Autodesk Inventor part; units mm, degrees
ref_plane "YZ Plane" through (0, 0, 0) normal (1, 0, 0) x (0, 1, 0)
ref_plane "XZ Plane" through (0, 0, 0) normal (0, 1, 0) x (-1, 0, 0)
ref_plane "XY Plane" through (0, 0, 0) normal (0, 0, 1) x (1, 0, 0)
sketch "Эскиз1" plane through (0, 0, 0) normal (0, 0, 1) x (1, 0, 0)
  line L0 (-8.89, 0) -> (53.01, 0)
  line L1 (53.01, 0) -> (53.01, 35.55)
  line L2 (53.01, 35.55) -> (-8.89, 35.55)
  line L3 (-8.89, 35.55) -> (-8.89, 0)
  circle A0 centre (15.24, 22.86) radius 0.405
  circle A1 centre (17.78, 22.86) radius 0.405
  circle A2 centre (20.32, 22.86) radius 0.405
  circle A3 centre (22.86, 22.86) radius 0.405
  circle A4 centre (25.4, 22.86) radius 0.405
  circle A5 centre (27.94, 22.86) radius 0.405
  circle A6 centre (37.62, 19.41) radius 0.405
  circle A7 centre (40.16, 19.41) radius 0.405
  circle A8 centre (0.1, 31.17) radius 0.65
  circle A9 centre (-4.9, 31.17) radius 0.65
  circle A10 centre (1.27, 20.32) radius 0.51
  circle A11 centre (-1.27, 20.32) radius 0.51
  circle A12 centre (-3.81, 20.32) radius 0.51
  circle A13 centre (-6.35, 20.32) radius 0.51
  circle A14 centre (48.26, 25.4) radius 0.65
  circle A15 centre (48.26, 30.4) radius 0.65
  circle A16 centre (9.33, 4.16) radius 0.51
  circle A17 centre (11.87, 4.16) radius 0.51
  circle A18 centre (14.41, 4.16) radius 0.51
  circle A19 centre (16.95, 4.16) radius 0.51
  circle A20 centre (19.49, 4.16) radius 0.51
  circle A21 centre (39.37, 15.24) radius 0.51
  circle A22 centre (41.91, 15.24) radius 0.51
  circle A23 centre (49.59, 7.57) radius 0.65
  circle A24 centre (49.59, 12.57) radius 0.65
  circle A25 centre (46.2, 8.43) radius 0.7
  circle A26 centre (46.2, 11.93) radius 0.7
  circle A27 centre (12.7, 24.13) radius 0.3
  circle A28 centre (5.08, 26.67) radius 0.3
  circle A29 centre (5.08, 24.13) radius 0.3
  circle A30 centre (12.7, 26.67) radius 0.3
  circle A31 centre (5.08, 31.75) radius 0.3
  circle A32 centre (5.08, 29.21) radius 0.3
  circle A33 centre (12.7, 29.21) radius 0.3
  circle A34 centre (12.7, 31.75) radius 0.3
  circle A35 centre (33.02, 25.4) radius 0.5
  circle A36 centre (33.02, 27.94) radius 0.5
  circle A37 centre (33.02, 22.86) radius 0.5
  circle A38 centre (-5.9225, 7.3465) radius 1.5
  circle A39 centre (39.37, 2.54) radius 1.5
  circle A40 centre (46.99, 19.05) radius 1.5
  circle A41 centre (6.0563, 20.3433) radius 1.5
  circle A42 centre (17.1236, 18.9948) radius 0.4
  circle A43 centre (17.0778, 15.6995) radius 0.4
extrude "OmniBot_motor_driver.brdКонтур" add sketch "Эскиз1" along normal blind 1.6
properties part number "000.006.001 - Плата"
Read the model definition and answer for the solid it produces. Units are mm, in the model's axes. Give positions to 0.01 mm unless a question says otherwise; leave off trailing zeros. Write each loop counter-clockwise with the first axis right and the second up, starting at its lowest first coordinate (ties: lowest second). Pieces come first, ordered by that corner, then holes. Notation, with made-up numbers: M -26,-18 L 14,-18 A10 cw 14,-8 Z; hole C -19,16.5 d11. An arc over 180 degrees is marked long. Put each result on its own line as item: value. Start each with the question number.
1. Consider line 1 along Y through (x, z) = (12.7, 0.9); line 2 along Y through (x, z) = (49.5, 0.95); line 3 along Y through (x, z) = (37.62, 1.15) (3 decimals). Determine where each line is inside the solid, lowest interval first.
2. For a pull along X with two mould halves and no side action, classify faces 1 (the cylindrical face through (48.42, 18.6, 0.79)), 2 (the flat face through (-8.89, 18, 1)), 3 (the flat face through (22, 18, 0)) as released by +X, released by -X, zero draft, split by the parting line, or undercut.
3. The part is cut by section A-A, the plane x = 0.1. Give the vertices of the cut face in (y, z), and give its area (3 significant figures).
4. This flat-tipped pin is pushed along its axis until it touches: pin 1 Ø2 at (x, y) = (46.2, 11.93) entering from +Z. Where does it stop, or does it pass through?
5. The part is cut by section B-B, the plane z = 0.95. Give the number of separate pieces and of enclosed holes in the cut face, and give its area (3 significant figures).
Final values:
1. line 1: y = 0 to 23.83, 24.43 to 26.37, 26.97 to 28.91, 29.51 to 31.45, 32.05 to 35.55
1. line 2: y = 0 to 6.93, 8.21 to 11.93, 13.21 to 35.55
1. line 3: y = 0 to 19.005, 19.815 to 35.55
2. face 1: undercut
2. face 2: released by -X
2. face 3: zero draft
3. outline: M 0,0 L 30.52,0 L 30.52,1.6 L 0,1.6 Z; M 31.82,0 L 35.55,0 L 35.55,1.6 L 31.82,1.6 Z
3. area: 54.8 mm²
4. pin 1: stops at z = 1.6
5. separate pieces: 1
5. enclosed holes: 44
5. area: 2,140 mm²
